Source: CAD feature listing. Evaluate the final solid. Frame: model axes, mm. Round coordinates to 2 decimals unless told otherwise and drop trailing zeros. Loops run counter-clockwise (first coordinate to the right, second up) from the corner with the lowest first, then second, coordinate; pieces in that order, holes last. Notation, with made-up numbers: (34.5, -25) - (49.5, -25) arc R19 cw to (49.5, -13) - close; hole circle Ø8 at (41, 68). An arc over 180 degrees is marked (long way). One line per question, with ' | ' between items.
from build123d import *

# Parameters (mm, degrees)
F0_R        = 16
F1_DEPTH    = 280
F2_W        = 45
F2_H        = 30
F3_DEPTH    = 4
F4_R        = 1.5
F5_DEPTH    = 25
F6_T1_DEPTH = 58
F6_T3_DEPTH = 57.9848728082
F7_R        = 1
F9_DEPTH    = 5


# Not quite as in the source:
# - a fillet or chamfer that OpenCascade refuses, or shapes differently, is made with other operations: its cross-section is extruded or revolved along the edge and cut away or added


with BuildPart() as f1:
    # F0 (on Top) → F1 (new body)
    with BuildSketch(Plane.XY):
        Circle(F0_R)
    extrude(amount=F1_DEPTH)

    # F2 (on Right) → F3 (join, symmetric)
    with BuildSketch(Plane.YZ):
        with Locations((22.5, 15)):
            Rectangle(F2_W, F2_H)
    extrude(amount=F3_DEPTH, both=True)

    # F4 (on face) → F5 (cut)
    with BuildSketch(Plane.YZ.offset(4)):
        with BuildLine():
            ThreePointArc((25.2459666924, 15), (30.2459666924, 10), (35.2459666924, 15))
            ThreePointArc((35.2459666924, 15), (30.2459666924, 20), (25.2459666924, 15))
        make_face()
        with BuildLine():
            ThreePointArc((-3.5, 286.5642011166), (0, 283.0642011166), (3.5, 286.5642011166))
            ThreePointArc((3.5, 286.5642011166), (0, 290.0642011166), (-3.5, 286.5642011166))
        make_face()
        with Locations((0, 286.5642011166)):
            Circle(F4_R, mode=Mode.SUBTRACT)
        with BuildLine():
            Line((3.5, 279.5200645924), (3.5, 286.5642011166))
            ThreePointArc((3.5, 286.5642011166), (0, 283.0642011166), (-3.5, 286.5642011166))
            Line((-3.5, 286.5642011166), (-3.5, 279.665210771))
            Line((-3.5, 279.665210771), (3.5, 279.5200645924))
        make_face()
        with BuildLine():
            Line((35.2459666924, 0), (35.2459666924, 15))
            ThreePointArc((35.2459666924, 15), (30.2459666924, 10), (25.2459666924, 15))
            Line((25.2459666924, 15), (25.2459666924, 0))
            Line((25.2459666924, 0), (35.2459666924, 0))
        make_face()
    extrude(amount=-F5_DEPTH, mode=Mode.SUBTRACT)

    # F6: fillet of radius 10 on 2 edges, made by hand

    # F6_s2 → F6_t1 (cut)
    with BuildSketch(Plane.YZ.offset(-29)):
        with BuildLine():
            ThreePointArc((35, 30), (42.0710678119, 27.0710678119), (45, 20))
            Line((45, 20), (45, 30))
            Line((45, 30), (35, 30))
        make_face()
    extrude(amount=F6_T1_DEPTH, mode=Mode.SUBTRACT)

    # F6_s4 → F6_t3 (cut)
    with BuildSketch(Plane.YZ.offset(-28.9924364041)):
        with BuildLine():
            ThreePointArc((35.2459666924, 0), (42.1575019009, 3.0134105333), (45, 9.9969745616))
            Line((45, 9.9969745616), (45, 0))
            Line((45, 0), (35.2459666924, 0))
        make_face()
    extrude(amount=F6_T3_DEPTH, mode=Mode.SUBTRACT)

    # F7
    f7_edges = [f1.edges().sort_by_distance(p)[0] for p in [
        (4, 42.071068, 27.071068),
        (-4, 45, 14.998487),
        (4, 35.245967, 7.5),
        (4, 30.245967, 20),
        (4, 25.245967, 7.5),
        (4, 20.36895, 0),
        (4, 15.491933, 15),
        (4, 25.245967, 30),
        (4, 45, 14.998487),
        (4, 42.157502, 3.013411),
        (12.649111, 9.797959, 0),
        (0, 16, 30),
        (-4, 15.491933, 15),
        (-9.797959, -12.649111, 0),
        (-4, 20.36895, 0),
        (-4, 25.245967, 30),
        (-4, 42.071068, 27.071068),
        (-4, 42.157502, 3.013411),
    ]]
    fillet(f7_edges, radius=F7_R)

    # F8 (on face) → F9 (join)
    with BuildSketch(Plane(origin=(-4, 0, 0), x_dir=(0, -1, 0), z_dir=(-1, 0, 0))):
        with BuildLine():
            Line((-3.1555609312, 289.529184103), (-3.1555609312, 279.529184103))
            Line((-3.1555609312, 279.529184103), (3.8444390688, 279.529184103))
            Line((3.8444390688, 279.529184103), (3.8444390688, 289.529184103))
            ThreePointArc((3.8444390688, 289.529184103), (0.3444390688, 286.029184103), (-3.1555609312, 289.529184103))
        make_face()
        with BuildLine():
            ThreePointArc((3.8444390688, 289.529184103), (0.3444390688, 293.029184103), (-3.1555609312, 289.529184103))
            Line((-3.1555609312, 289.529184103), (-1.1555609312, 289.529184103))
            ThreePointArc((-1.1555609312, 289.529184103), (0.3444390688, 291.029184103), (1.8444390688, 289.529184103))
            Line((1.8444390688, 289.529184103), (3.8444390688, 289.529184103))
        make_face()
        with BuildLine():
            Line((-1.1555609312, 289.529184103), (-3.1555609312, 289.529184103))
            ThreePointArc((-3.1555609312, 289.529184103), (0.3444390688, 286.029184103), (3.8444390688, 289.529184103))
            Line((3.8444390688, 289.529184103), (1.8444390688, 289.529184103))
            ThreePointArc((1.8444390688, 289.529184103), (0.3444390688, 288.029184103), (-1.1555609312, 289.529184103))
        make_face()
    extrude(amount=-F9_DEPTH)


solid = f1.part
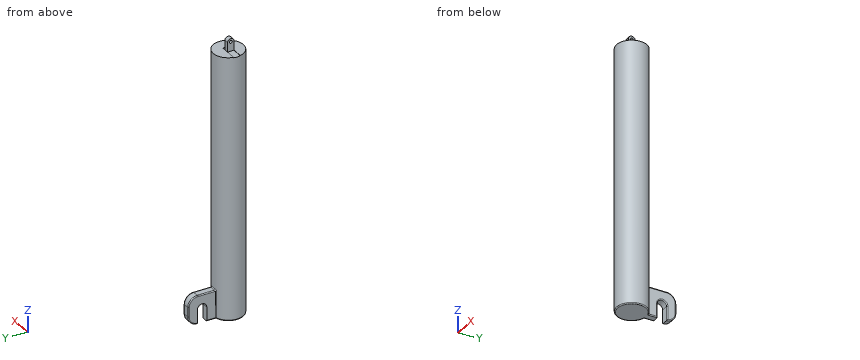
1. Material intervals for probe 1 along Y at (x, z) = (1, 168); probe 2 along Z at (x, y) = (-13.5, -2); probe 3 along X at (y, z) = (42, 22), sorted ascending.
Worked out:
probe 1: y = -15.97 to 15.97 | probe 2: z = 0 to 279.63 | probe 3: x = -4 to 4
2. Contact query for flat-ended pins moving along their axis: P1, Ø1.5, axis at x = 6.5, z = 232, coming from the +Y side; P2, Ø1.8, axis at x = 0.5, y = 30, coming from the +Z side; P3, Ø3.5, axis at y = -1.5, z = 286, coming from the -X side; P4, Ø10, axis at y = 22, z = 53, coming from the -X side. Output: stop coordinate, or through.
Worked out:
P1: stops at y = 14.93 | P2: stops at z = 30 | P3: stops at x = -4 | P4: passes through
3. Section query A-A, the plane z = 262.5. Return loops of the section in (x, y).
Worked out:
outline: circle Ø32 at (0, 0)
